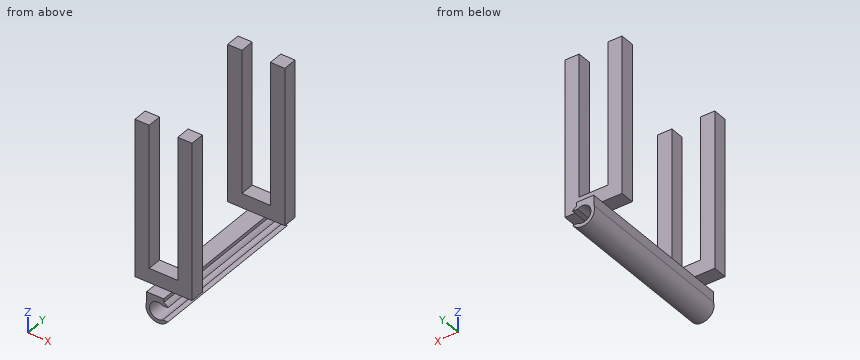
```python
from build123d import *

# Parameters (mm, degrees)
F1_DEPTH = 73.66
F3_DEPTH = 73.66
F4_W     = 25.4
F4_H     = 6.349999
F4_H_2   = 6.35
F5_DEPTH = 69.85
F6_W     = 12.7
F6_H     = 63.5
F7_DEPTH = 63.5


with BuildPart() as f1:
    # F0 (on Front) → F1 (new body)
    with BuildSketch(Plane.XZ):
        with BuildLine():
            ThreePointArc((2.106057, -3.175), (-3.81, 0), (2.106057, 3.175))
            Line((2.106057, 3.175), (4.364903, 3.175))
            ThreePointArc((4.364903, 3.175), (-5.3975, 0), (4.364903, -3.175))
            Line((4.364903, -3.175), (2.106057, -3.175))
        make_face()
    extrude(amount=F1_DEPTH)

    # F2 (on face) → F3 (join, through all)
    with BuildSketch(Plane.XZ.offset(73.66)):
        with BuildLine():
            Line((-5.08, 6.35), (-5.08, 1.823899))
            ThreePointArc((-5.08, 1.823899), (-1.942098, 5.035997), (2.54, 4.7625))
            Line((2.54, 4.7625), (2.54, 6.35))
            Line((2.54, 6.35), (-5.08, 6.35))
        make_face()
    extrude(amount=-F3_DEPTH)

    # F4 (on face) → F5 (join)
    with BuildSketch(Plane.XY.offset(6.35)):
        with Locations((-1.27, -65.405)):
            Rectangle(F4_W, F4_H)
        with Locations((-1.27, -8.255)):
            Rectangle(F4_W, F4_H_2)
    extrude(amount=F5_DEPTH)

    # F6 (on face) → F7 (cut, through all)
    with BuildSketch(Plane.XZ.offset(68.58)):
        with Locations((-1.27, 44.45)):
            Rectangle(F6_W, F6_H)
    extrude(amount=-F7_DEPTH, mode=Mode.SUBTRACT)


solid = f1.part
```
Verification items for the finished model (mm, model axes). Give positions to 0.01 mm unless a question says otherwise; leave off trailing zeros. Order: outer loops, then holes, each group sorted by start corner. A loop starts at its lowest first (then second) coordinate and runs counter-clockwise, first axis right, second up. Notation, with made-up numbers: M 3,-2 L 34,-2 A26 ccw 34,36 Z; hole C -32.5,58.5 d9. An arc over 180 degrees is marked long. Answer in a Markdown table with one row per item. Add a question column.
Item 1: Gauge pin test, flat ends, axial feed: pin 1 (1.5 mm diameter, centred on x = 0.5, y = -72, fed in from +Z); pin 2 (1.5 mm diameter, centred on x = 0, y = -12, fed in from +Z); pin 3 (0.7 mm diameter, centred on x = 3, y = -26.5, fed in from -Z); pin 4 (6 mm diameter, centred on y = -16, z = 28.5, fed in from +X). Record the tip position at first contact, or that the pin passes through.
Item 2: Section check C-C, the plane z = 10. Enter the section's corners in (x, y), and give its area (3 significant figures).
Item 3: Section check B-B, the plane z = 41. Enter the section's corners in (x, y).
Item 4: Section check A-A, the plane x = 0. Enter the section's corners in (y, z), and give its area (3 significant figures).
Item 5: Scan lines: probe 1 along Y at (x, z) = (-13, 26); probe 2 along X at (y, z) = (-6, 32); probe 3 along Z at (x, y) = (0, -44). Record each from-to range of solid material in increasing order. Write a range as from..to.
Filled sheet:
| question | item | result |
|---|---|---|
| 1 | pin 1 | stops at z = 6.35 |
| 1 | pin 2 | stops at z = 12.7 |
| 1 | pin 3 | stops at z = -4.7 |
| 1 | pin 4 | passes through |
| 2 | outline | M -13.97,-68.58 L 11.43,-68.58 L 11.43,-62.23 L -13.97,-62.23 Z; M -13.97,-11.43 L 11.43,-11.43 L 11.43,-5.08 L -13.97,-5.08 Z |
| 2 | area | 323 mm^2 |
| 3 | outline | M -13.97,-68.58 L -7.62,-68.58 L -7.62,-62.23 L -13.97,-62.23 Z; M -13.97,-11.43 L -7.62,-11.43 L -7.62,-5.08 L -13.97,-5.08 Z; M 5.08,-68.58 L 11.43,-68.58 L 11.43,-62.23 L 5.08,-62.23 Z; M 5.08,-11.43 L 11.43,-11.43 L 11.43,-5.08 L 5.08,-5.08 Z |
| 4 | outline | M -73.66,-5.4 L 0,-5.4 L 0,-3.81 L -73.66,-3.81 Z; M -73.66,3.81 L 0,3.81 L 0,6.35 L -5.08,6.35 L -5.08,12.7 L -11.43,12.7 L -11.43,6.35 L -62.23,6.35 L -62.23,12.7 L -68.58,12.7 L -68.58,6.35 L -73.66,6.35 Z |
| 4 | area | 385 mm^2 |
| 5 | probe 1 | y = -68.58..-62.23, -11.43..-5.08 |
| 5 | probe 2 | x = -13.97..-7.62, 5.08..11.43 |
| 5 | probe 3 | z = -5.4..-3.81, 3.81..6.35 |
